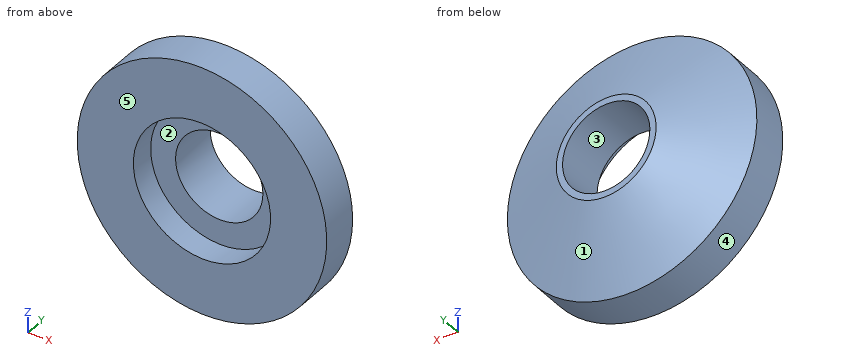
from build123d import *

# Parameters (mm, degrees)
CROQUIS1_R              = 50
SALIENTE_EXTRUIR1_DEPTH = 15
CROQUIS3_R              = 20
CROQUIS4_R              = 17.5
CORTAR_EXTRUIR1_DEPTH   = 77.811457609
CROQUIS5_R              = 27.5
CORTAR_EXTRUIR2_DEPTH   = 10


with BuildPart() as part:
    # Croquis1 → Saliente-Extruir1 (new body)
    with BuildSketch(Plane(origin=(0, 0, 0), x_dir=(1, 0, 0), z_dir=(0, 1, 0))):
        with Locations(Location((0, 0, 0), (0, 0, 270))):
            Circle(CROQUIS1_R)
    extrude(amount=SALIENTE_EXTRUIR1_DEPTH)

    # Croquis3 → section 0 of recubrir1
    with BuildSketch(Plane(origin=(0, 30, 0), x_dir=(1, 0, 0), z_dir=(0, 1, 0)), mode=Mode.PRIVATE) as recubrir1_s0:
        Circle(CROQUIS3_R)
    # loft up to a face of the part (recubrir1)
    loft([recubrir1_s0.sketch, Face(Wire([part.edges().sort_by_distance((36.448431371, 15, -34.227355296))[0]]))])

    # Croquis4 → Cortar-Extruir1 (cut, through all)
    with BuildSketch(Plane(origin=(0, 30, 0), x_dir=(1, 0, 0), z_dir=(0, 1, 0))):
        with Locations(Location((0, 0, 0), (0, 0, 270))):
            Circle(CROQUIS4_R)
    extrude(amount=-CORTAR_EXTRUIR1_DEPTH, mode=Mode.SUBTRACT)

    # Croquis5 → Cortar-Extruir2 (cut)
    with BuildSketch(Plane.XZ):
        with Locations(Location((0, 0, 0), (0, 0, 270))):
            Circle(CROQUIS5_R)
    extrude(amount=-CORTAR_EXTRUIR2_DEPTH, mode=Mode.SUBTRACT)


solid = part.part
Build history of the part. All positions in model axes, mm. Face numbers are marked on the shaded views. A direction names the side the tool comes from. Coordinates: 2 decimals unless noted, no trailing zeros. Order: outer loops, then holes, each group sorted by start corner. A loop starts at its lowest first (then second) coordinate and runs counter-clockwise, first axis right, second up. Notation, with made-up numbers: (64.25, 5) - (80.25, 5) arc R26 cw to (80.25, 42) - close; hole circle Ø8 at (9, 3.25). An arc over 180 degrees is marked (long way). Write item = value, one per line. Start each with the question number.
1) Two-plate mould, pull along Z, no slides. Class the marked faces 3, 4 and 5: pulls with the +Z half, pulls with the -Z half, needs draft (parallel to the pull), parting line crosses it, or undercut.
2) Flat gauge pins, fed straight in: pin 1 Ø1.5 at (x, y) = (-24.5, 17) entering from +Z; pin 2 Ø2 at (y, z) = (3, -30.5) entering from -X; pin 3 Ø8 at (x, z) = (-1, -27.5) entering from +Y. Where does each tip first touch, or does it go through?
3) 3-axis set-ups, long thin cutter, end or side, ignore diameter. For the marked faces 1 and 2: which of +Z, -Z, +X, -X, +Y, -Y reach the whole face in a straight line?
4) Saw through at A-A on x = 0. Write the cut outline in (y, z).
5) Wall check: line 1 along X through (y, z) = (6.25, 0); line 2 along Z through (x, y) = (-10.5, 12); line 3 along Z through (x, y) = (0.5, 23). Give the ranges that are in metal, low to high. Write a range as from..to.
6) Saw through at B-B on y = 17.5. Write the cut outline in (x, z).
From the geometry:
q1.face_3 = undercut
q1.face_4 = parting line crosses it
q1.face_5 = needs draft
q2.pin_1 = 40.75
q2.pin_2 = -40.37
q2.pin_3 = 28.24
q3.face_1 = +Y
q3.face_2 = -Y
q4.outline = (0, -50) - (15, -50) - (30, -20) - (30, -17.5) - (10, -17.5) - (10, -27.5) - (0, -27.5) - close; (0, 27.5) - (10, 27.5) - (10, 17.5) - (30, 17.5) - (30, 20) - (15, 50) - (0, 50) - close
q5.line_1 = -50..-27.5, 27.5..50
q5.line_2 = -48.89..-14, 14..48.89
q5.line_3 = -34..-17.49, 17.49..34
q6.outline = circle Ø90 at (0, 0); hole circle Ø35 at (0, 0)
